For this review, take the finished solid that the model builds, in its own axes (mm). Face numbers are marked on the shaded views. A direction names the side the tool comes from. Coordinates: 2 decimals unless noted, no trailing zeros. Order: outer loops, then holes, each group sorted by start corner. A loop starts at its lowest first (then second) coordinate and runs counter-clockwise, first axis right, second up. Notation, with made-up numbers: (6, 67) -> (23, 67) arc R20 cw to (23, 104) -> close; hole circle Ø8 at (59, 50). An arc over 180 degrees is marked (long way). Return JSON: item names as keys, results as strings. Group by question number.
Item 1: Draft analysis for pull direction X (two halves, no side actions). For the marked faces 1, 2, 3 and 4, state which applies: +X half, -X half, draft (parallel to the pull), parting line (faces both ways), or undercut.
Item 2: Insertion check: pin 1 (4 mm diameter, centred on y = 6, z = 7.5, fed in from +X); pin 2 (8 mm diameter, centred on x = 9, y = 9, fed in from +Z); pin 3 (5 mm diameter, centred on y = 21.5, z = 2, fed in from -X); pin 4 (12 mm diameter, centred on x = 2, y = 1.5, fed in from -Z). Each pin has a flat end and moves straight along its axis. Give the tip position at first contact, or say it passes through.
Item 3: Take a section at D-D (x = 16.5). Write out the cut boundary in (y, z).
Item 4: For line 1 along Y through (x, z) = (0, 8.25) (3 decimals); line 2 along X through (y, z) = (0, 5.5) (3 decimals); line 3 along Z through (x, y) = (-6, -12.5), list the stretches that pass through material, from the lowest coordinate up.
Item 5: Take a section at B-B (z = 8.25). Write out the cut boundary in (x, y) (3 decimals), then the cut area to 3 significant figures.
Item 6: Machinability: for the marked faces 5 and 6, which of the approach directions +Z, -Z, +X, -X, +Y, -Y give a long, thin tool a straight path to every point of the face, cutting with its end or side? Answer none if there is none.
Item 7: Take a section at C-C (y = 29). Write out the cut boundary in (x, z), then the cut area to 3 significant figures.
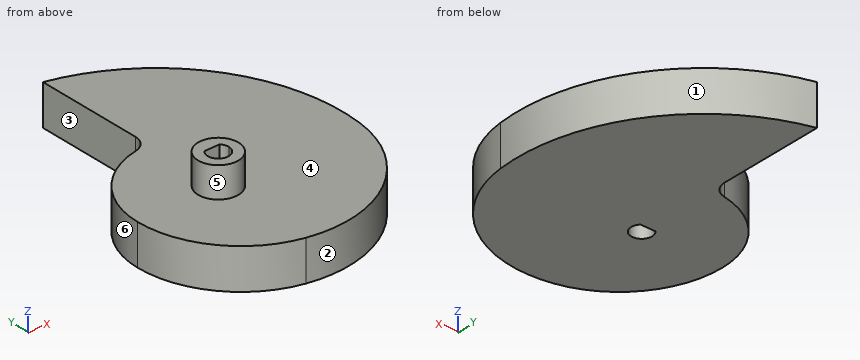
```python
from build123d import *

# Parameters (mm, degrees)
BOSS_EXTRUDE1_DEPTH = 6.35
SKETCH2_R           = 3.175
BOSS_EXTRUDE2_DEPTH = 4.7625
CUT_EXTRUDE1_DEPTH  = 12.1125
FILLET1_R           = 2.54


with BuildPart() as part:
    # Sketch1 → Boss-Extrude1 (new body)
    with BuildSketch(Plane.XY):
        with BuildLine():
            ThreePointArc((0, -15.875), (14.664616841, -12.910463577), (22.225, 0))
            ThreePointArc((22.225, 0), (17.085257234, 20.055930064), (0, 31.75))
            Line((0, 31.75), (0, 0))
            Line((0, 0), (-12.7, 0))
            ThreePointArc((-12.7, 0), (-9.134324659, -10.164959727), (0, -15.875))
        make_face()
        with BuildLine():
            Line((-12.7, 0), (0, 0))
            Line((0, 0), (0, 12.7))
            ThreePointArc((0, 12.7), (-8.980256121, 8.980256121), (-12.7, 0))
        make_face()
    extrude(amount=BOSS_EXTRUDE1_DEPTH)

    # Sketch2 → Boss-Extrude2 (add)
    with BuildSketch(Plane.XY.offset(6.35)):
        Circle(SKETCH2_R)
    extrude(amount=BOSS_EXTRUDE2_DEPTH)

    # Sketch3 → Cut-Extrude1 (cut, through all)
    with BuildSketch(Plane.XY.offset(11.1125)):
        with BuildLine():
            Line((1.191365603, 1.143), (-1.191365603, 1.143))
            ThreePointArc((-1.191365603, 1.143), (-0.61597743, -1.531787454), (1.651, 0))
            ThreePointArc((1.651, 0), (1.531787454, 0.61597743), (1.191365603, 1.143))
        make_face()
    extrude(amount=-CUT_EXTRUDE1_DEPTH, mode=Mode.SUBTRACT)

    # Fillet1
    fillet1_edges = [part.edges().sort_by_distance(p)[0] for p in [
        (0, 12.7, 3.175),
    ]]
    fillet(fillet1_edges, radius=FILLET1_R)


solid = part.part
```
Findings below:
{
 "1": {"face 1": "+X half", "face 2": "parting line", "face 3": "-X half", "face 4": "draft"},
 "2": {"pin 1": "stops at x = 22.38", "pin 2": "stops at z = 6.35", "pin 3": "stops at x = 0", "pin 4": "stops at z = 0"},
 "3": {"outline": "(-11.41, 0) -> (20.86, 0) -> (20.86, 6.35) -> (-11.41, 6.35) -> close"},
 "4": {"line 1": "y = -3.175 to -1.651, 1.143 to 3.175", "line 2": "x = -12.7 to -1.651, 1.651 to 22.225", "line 3": "z = 0 to 6.35"},
 "5": {"outline": "circle Ø6.35 at (0, 0); hole (-1.191, 1.143) arc R1.651 ccw (long way) to (1.191, 1.143) -> close", "area": "23.9 mm2"},
 "6": {"face 5": "+Z", "face 6": "+Z, -Z, -X, +Y"},
 "7": {"outline": "(0, 0) -> (7.09, 0) -> (7.09, 6.35) -> (0, 6.35) -> close", "area": "45.0 mm2"}
}
